Geometry check sheet. Reference: the model listing, model coordinates, mm. Face numbers are marked on the shaded views. A direction names the side the tool comes from. Coordinates: 2 decimals unless noted, no trailing zeros. Order: outer loops, then holes, each group sorted by start corner. A loop starts at its lowest first (then second) coordinate and runs counter-clockwise, first axis right, second up. Notation, with made-up numbers: (77.5, -24.5) -> (94.5, -24.5) arc R25 ccw to (94.5, -9.5) -> close; hole circle Ø2 at (-40, 75). An arc over 180 degrees is marked (long way). Answer in a Markdown table with one row per item. Add a question column.
```python
from build123d import *

# Parameters (mm, degrees)
BOSS_EXTRUDE1_DEPTH      = 5
BOSS_EXTRUDE3_START      = 5
SKETCH1_5_R              = 4
BOSS_EXTRUDE3_DEPTH      = 5.75
BOSS_EXTRUDE2_START      = 10.75
SKETCH1_4_R              = 3.125
BOSS_EXTRUDE2_DEPTH      = 5.25
BOSS_EXTRUDE4_START      = 5
SKETCH1_6_R              = 4.25
BOSS_EXTRUDE4_DEPTH      = 29.85
BOSS_EXTRUDE5_DEPTH      = 2.25
BOSS_EXTRUDE6_DEPTH      = 29.85
FILLET1_R                = 1
M2_5X0_45_TAPPED_HOLE1_D = 2.05
CHAMFER1_SIZE            = 1


# Read off the part's stored shape, not the designer's step: Boss-Extrude5
with BuildPart() as part:
    # Sketch1 → Boss-Extrude1 (new body)
    with BuildSketch(Plane.XY):
        with BuildLine():
            ThreePointArc((3.999567451, 32.058823529), (0, 36), (-3.999567451, 32.058823529))
            Line((-3.999567451, 32.058823529), (-4.470104798, 0.065743945))
            ThreePointArc((-4.470104798, 0.065743945), (0, -4.470588235), (4.470104798, 0.065743945))
            Line((4.470104798, 0.065743945), (3.999567451, 32.058823529))
        make_face()
    extrude(amount=BOSS_EXTRUDE1_DEPTH)

    # Sketch1<5> → Boss-Extrude3 (add)
    with BuildSketch(Plane.XY.offset(BOSS_EXTRUDE3_START)):
        with Locations(Location((0, 32, 0), (0, 0, 179.157384634))):
            Circle(SKETCH1_5_R)
    extrude(amount=BOSS_EXTRUDE3_DEPTH)

    # Sketch1<4> → Boss-Extrude2 (add)
    with BuildSketch(Plane.XY.offset(BOSS_EXTRUDE2_START)):
        with Locations(Location((0, 32, 0), (0, 0, 180))):
            Circle(SKETCH1_4_R)
    extrude(amount=BOSS_EXTRUDE2_DEPTH)

    # Sketch1<6> → Boss-Extrude4 (add)
    with BuildSketch(Plane.XY.offset(BOSS_EXTRUDE4_START)):
        Circle(SKETCH1_6_R)
        with Locations(Location((0, 15, 0), (0, 0, 179.157384634))):
            Circle(SKETCH1_6_R)
    extrude(amount=BOSS_EXTRUDE4_DEPTH)

    # Boss-Extrude5 outline → Boss-Extrude5 (add)
    with BuildSketch(Plane.XY.offset(5)):
        with BuildLine():
            Line((-4.249540417, 15.06249996), (-4.470104798, 0.065743945))
            ThreePointArc((-4.470104798, 0.065743945), (0, -4.470588235), (4.470104798, 0.065743945))
            Line((4.470104798, 0.065743945), (4.249540416, 15.062500001))
            ThreePointArc((4.249540416, 15.062500001), (3.35933087, 12.396656745), (1, 10.86932209))
            Line((1, 10.86932209), (1, 4.13067791))
            ThreePointArc((1, 4.13067791), (0, -4.25), (-1, 4.13067791))
            Line((-1, 4.13067791), (-1, 10.86932209))
            ThreePointArc((-1, 10.86932209), (-3.359330858, 12.396656729), (-4.249540417, 15.06249996))
        make_face()
        with BuildLine():
            Line((-3.999567451, 32.058823529), (-4.249540417, 15.06249996))
            ThreePointArc((-4.249540417, 15.06249996), (-3.320683154, 17.652463646), (-1, 19.13067791))
            Line((-1, 19.13067791), (-1, 28.127016654))
            ThreePointArc((-1, 28.127016654), (-3.18020361, 29.573829149), (-3.999567451, 32.058823529))
        make_face()
        with BuildLine():
            ThreePointArc((1, 19.13067791), (3.320683141, 17.652463662), (4.249540416, 15.062500001))
            Line((4.249540416, 15.062500001), (3.999567451, 32.058823529))
            ThreePointArc((3.999567451, 32.058823529), (3.18020361, 29.573829149), (1, 28.127016654))
            Line((1, 28.127016654), (1, 19.13067791))
        make_face()
    extrude(amount=BOSS_EXTRUDE5_DEPTH)

    # Sketch2<3> → Boss-Extrude6 (add)
    with BuildSketch(Plane.XY.offset(5)):
        with BuildLine():
            ThreePointArc((1, 10.86932209), (0, 10.75), (-1, 10.86932209))
            Line((-1, 10.86932209), (-1, 4.13067791))
            ThreePointArc((-1, 4.13067791), (0, 4.25), (1, 4.13067791))
            Line((1, 4.13067791), (1, 10.86932209))
        make_face()
    extrude(amount=BOSS_EXTRUDE6_DEPTH)

    # Fillet1
    fillet1_edges = [part.edges().sort_by_distance(p)[0] for p in [
        (1, 4.13067791, 21.05),
        (1, 10.86932209, 21.05),
        (-1, 4.13067791, 21.05),
        (-1, 10.86932209, 21.05),
        (-1, 28.127016654, 6.125),
        (1, 28.127016654, 6.125),
        (-1, 19.13067791, 6.125),
        (1, 19.13067791, 6.125),
    ]]
    fillet(fillet1_edges, radius=FILLET1_R - 0.0001)  # a hair under: the kernel refuses the full size

    # M2.5x0.45 Tapped Hole1 (through all)
    with Locations(Plane.XY.offset(34.85)):
        with Locations((0, 15), (0, 0), (0, 32)):
            Hole(M2_5X0_45_TAPPED_HOLE1_D / 2)

    # Chamfer1
    chamfer1_edges = [part.edges().sort_by_distance(p)[0] for p in [
        (3.125, 32, 16),
    ]]
    chamfer(chamfer1_edges, length=CHAMFER1_SIZE)


solid = part.part
```
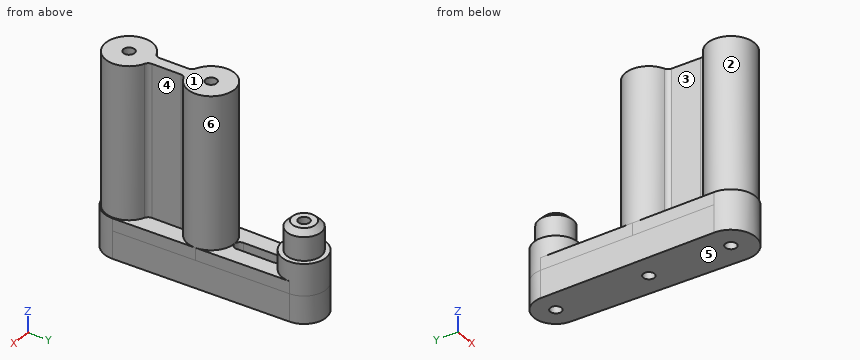
(1) Cross-section at A-A (z = 23). Enter the section's corners in (x, y) (3 decimals).
(2) Mould release check, pull along Y, two halves, no side actions. Record for the marked faces 1 and 2: +Y half, -Y half, draft (parallel to the pull), parting line (faces both ways), or undercut.
(3) Cross-section at C-C (y = 7.5). Enter the section's corners in (x, z), plus the area to 3 significant figures.
(4) Go/stop test with flat-tipped pins: P1, Ø2, axis at x = 3, y = 27.5, coming from the +Z side; P2, Ø1.5, axis at y = 9, z = 15.5, coming from the -X side; P3, Ø0.7, axis at y = 23, z = 6.5, coming from the +X side. Record where each tip stops, or that it passes through.
(5) Cross-section at B-B (y = 21). Enter the section's corners in (x, z), plus the area to 3 significant figures.
(6) Scan lines: line 1 along Y through (x, z) = (0, 22) (3 decimals); line 2 along Y through (x, z) = (0, 10) (3 decimals); line 3 along Z through (x, y) = (3.25, 6.5). Record each from-to range of solid material in increasing order.
(7) Access from +Z, -Z, +X, -X, +Y, -Y to the whole of each face (thin tool, end or side, straight path). Record for the marked faces 3, 4, 5 and 6.
Checks:
| question | item | result |
|---|---|---|
| 1 | outline | (-1.619, 3.93) arc R4.25 ccw (long way) to (1.619, 3.93) arc R1 cw to (1, 4.854) -> (1, 10.146) arc R1 cw to (1.619, 11.07) arc R4.25 ccw (long way) to (-1.619, 11.07) arc R1 cw to (-1, 10.146) -> (-1, 4.854) arc R1 cw to start; hole circle Ø2.05 at (0, 0); hole circle Ø2.05 at (0, 15) |
| 2 | face 1 | draft |
| 2 | face 2 | undercut |
| 3 | outline | (-4.36, 0) -> (4.36, 0) -> (4.36, 7.25) -> (1, 7.25) -> (1, 34.85) -> (-1, 34.85) -> (-1, 7.25) -> (-4.36, 7.25) -> close |
| 3 | area | 118 mm² |
| 4 | P1 | z = 7.25 |
| 4 | P2 | x = -1 |
| 4 | P3 | x = 4.14 |
| 5 | outline | (-4.16, 0) -> (4.16, 0) -> (4.16, 7.25) -> (1, 7.25) -> (1, 5) -> (-1, 5) -> (-1, 7.25) -> (-4.16, 7.25) -> close |
| 5 | area | 55.9 mm² |
| 6 | line 1 | -4.25 to -1.025, 1.025 to 13.975, 16.025 to 19.25 |
| 6 | line 2 | -4.25 to -1.025, 1.025 to 13.975, 16.025 to 19.25, 28 to 30.975, 33.025 to 36 |
| 6 | line 3 | 0 to 7.25 |
| 7 | face 3 | +Z, -X |
| 7 | face 4 | +Z, +X |
| 7 | face 5 | -Z, +X, -X, +Y, -Y |
| 7 | face 6 | +Z |
